Here's how the part is built. I have some questions about the finished solid (model axes, mm). Round coordinates to 2 decimals unless told otherwise and drop trailing zeros. Write each loop counter-clockwise with the first axis right and the second up, starting at its lowest first coordinate (ties: lowest second). Pieces come first, ordered by that corner, then holes. Notation, with made-up numbers: (-15, -26.5) - (-2, -26.5) arc R6 cw to (-2, -15.5) - close; hole circle Ø7 at (5.5, 46). An arc over 180 degrees is marked (long way). Return JSON: item names as keys, results as strings. Group by question number.
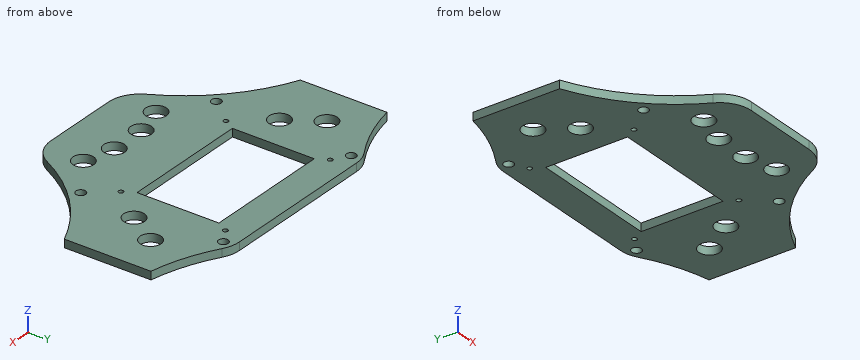
```python
from build123d import *

# Parameters (mm, degrees)
ESBO_O1_R                = 6.5
ESBO_O1_R_2              = 3
ESBO_O1_R_3              = 1.5
ESBO_O1_W                = 80
ESBO_O1_H                = 51
RESSALTO_EXTRUS_O1_DEPTH = 5


with BuildPart() as part:
    # Esboço1 → Ressalto-extrusão1 (new body)
    with BuildSketch(Plane.XY):
        with BuildLine():
            Line((-49.119135606, 68), (49.119135606, 68))
            ThreePointArc((49.119135606, 68), (54.543435225, 67.250375935), (59.56111629, 65.057697365))
            ThreePointArc((59.56111629, 65.057697365), (78.583692726, 55.703629757), (99, 50))
            Line((99, 50), (99, -4))
            ThreePointArc((99, -4), (65.800143376, -25.584477196), (41.890064111, -57.150728877))
            ThreePointArc((41.890064111, -57.150728877), (34.522230169, -65.073584532), (24.106246719, -68))
            Line((24.106246719, -68), (-24.106246719, -68))
            ThreePointArc((-24.106246719, -68), (-34.522230169, -65.073584532), (-41.890064111, -57.150728877))
            ThreePointArc((-41.890064111, -57.150728877), (-65.800143376, -25.584477196), (-99, -4))
            Line((-99, -4), (-99, 50))
            ThreePointArc((-99, 50), (-78.583692726, 55.703629757), (-59.56111629, 65.057697365))
            ThreePointArc((-59.56111629, 65.057697365), (-54.543435225, 67.250375935), (-49.119135606, 68))
        make_face()
        with Locations((74, 31.167626134)):
            Circle(ESBO_O1_R, mode=Mode.SUBTRACT)
        with Locations((61, 11.261041117)):
            Circle(ESBO_O1_R, mode=Mode.SUBTRACT)
        with Locations((11.289140568, -38)):
            Circle(ESBO_O1_R, mode=Mode.SUBTRACT)
        with Locations((30.514158569, -43)):
            Circle(ESBO_O1_R, mode=Mode.SUBTRACT)
        with Locations((-53.62430165, 61.446355775)):
            Circle(ESBO_O1_R_2, mode=Mode.SUBTRACT)
        with Locations((-56.834913612, -25.028841797)):
            Circle(ESBO_O1_R_2, mode=Mode.SUBTRACT)
        with Locations((-44, 55.5)):
            Circle(ESBO_O1_R_3, mode=Mode.SUBTRACT)
        with Locations((-44, -9.5)):
            Circle(ESBO_O1_R_3, mode=Mode.SUBTRACT)
        with Locations((44, -9.5)):
            Circle(ESBO_O1_R_3, mode=Mode.SUBTRACT)
        with Locations((44, 55.5)):
            Circle(ESBO_O1_R_3, mode=Mode.SUBTRACT)
        with Locations((56.834913612, -25.028841797)):
            Circle(ESBO_O1_R_2, mode=Mode.SUBTRACT)
        with Locations((-30.514158569, -43)):
            Circle(ESBO_O1_R, mode=Mode.SUBTRACT)
        with Locations((-11.289140568, -38)):
            Circle(ESBO_O1_R, mode=Mode.SUBTRACT)
        with Locations((-61, 11.261041117)):
            Circle(ESBO_O1_R, mode=Mode.SUBTRACT)
        with Locations((53.62430165, 61.446355775)):
            Circle(ESBO_O1_R_2, mode=Mode.SUBTRACT)
        with Locations((-74, 31.167626134)):
            Circle(ESBO_O1_R, mode=Mode.SUBTRACT)
        with Locations((0, 23)):
            Rectangle(ESBO_O1_W, ESBO_O1_H, mode=Mode.SUBTRACT)
    extrude(amount=RESSALTO_EXTRUS_O1_DEPTH)


solid = part.part
```
1) Imagine slicing it at D-D (z = 1.4). Give the number of separate pieces and of enclosed holes in the cut face, plus the area to 3 significant figures.
2) Imagine slicing it at C-C (y = 35). Please give me the cut outline in (x, z), plus the area to 3 significant figures.
3) Imagine slicing it at B-B (x = -73). Please give me the cut outline in (y, z) (3 decimals).
4) I need wall thicknesses on line 1 along X through (y, z) = (2, 3.75); line 2 along X through (y, z) = (-32.5, 4); line 3 along X through (y, z) = (-46, 4.35). Which ranges of each line are inside material? Lowest first, please.
5) Imagine slicing it at A-A (y = 0). Please give me the cut outline in (x, z), plus the area to 3 significant figures.
6) Will this pin go through, and if not, where does the flat tip stop? pin 1 Ø1.5 at (y, z) = (-30, 1.5) entering from +X.
Results found:
{
 "1": {"separate pieces": "1", "enclosed holes": "17", "area": "15,600 mm²"},
 "2": {"outline": "(-99, 0) - (-79.25, 0) - (-79.25, 5) - (-99, 5) - close; (-68.75, 0) - (-40, 0) - (-40, 5) - (-68.75, 5) - close; (40, 0) - (68.75, 0) - (68.75, 5) - (40, 5) - close; (79.25, 0) - (99, 0) - (99, 5) - (79.25, 5) - close", "area": "485 mm²"},
 "3": {"outline": "(-19.418, 0) - (24.745, 0) - (24.745, 5) - (-19.418, 5) - close; (37.59, 0) - (58.005, 0) - (58.005, 5) - (37.59, 5) - close"},
 "4": {"line 1": "x = -99 to -40, 40 to 99", "line 2": "x = -58.97 to -14.75, -7.83 to 7.83, 14.75 to 58.97", "line 3": "x = -48.45 to -36.28, -24.75 to 24.75, 36.28 to 48.45"},
 "5": {"outline": "(-99, 0) - (-40, 0) - (-40, 5) - (-99, 5) - close; (40, 0) - (99, 0) - (99, 5) - (40, 5) - close", "area": "590 mm²"},
 "6": {"pin 1": "stops at x = 62.04"}
}
